Here's how the part is built. I have some questions about the finished solid (model axes, mm). A direction names the side the tool comes from. Give positions to 0.01 mm unless a question says otherwise; leave off trailing zeros. Loops run counter-clockwise (first coordinate to the right, second up) from the corner with the lowest first, then second, coordinate; pieces in that order, holes last. Notation, with made-up numbers: (2.25, 85) - (24.25, 85) arc R11 ccw to (24.25, 106) - close; hole circle Ø3 at (-39, -27.75). An arc over 180 degrees is marked (long way). Use a Markdown table: item, result.
from build123d import *

# Parameters (mm, degrees)
F0_W     = 10
F0_H     = 10.8
F1_DEPTH = 10
F2_R     = 4
F3_DEPTH = 30
F4_R     = 2
F5_DEPTH = 25


with BuildPart() as f1:
    # F0 (on Right) → F1 (new body)
    with BuildSketch(Plane.YZ):
        with Locations((16.265796, 5.4)):
            Rectangle(F0_W, F0_H)
    extrude(amount=F1_DEPTH)

    # F2 (on face) → F3 (join)
    with BuildSketch(Plane.YZ.offset(10)):
        with Locations((16.265796, 5.4)):
            Circle(F2_R)
    extrude(amount=F3_DEPTH)

    # F4 (on face) → F5 (cut)
    with BuildSketch(Plane.XZ.offset(-11.265796)):
        with Locations((5, 5.4)):
            Circle(F4_R)
    extrude(amount=-F5_DEPTH, mode=Mode.SUBTRACT)


solid = f1.part
(1) If I drill on line 1 (Z direction, x = 5, y = 18.5); line 2 (X direction, y = 14.75, z = 5.5); line 3 (Z direction, x = 16.5, y = 16.25), over which ranges is the centre line in solid material (lowest first)?
A:
| item | result |
|---|---|
| line 1 | 0 to 3.4, 7.4 to 10.8 |
| line 2 | 0 to 3, 7 to 40 |
| line 3 | 1.4 to 9.4 |
(2) We'd pull the mould along Z, two halves only. Please class faces 3 (the face through (2.7, 11.266, 5.3)), 4 (the face through (24.79, 20.08, 6.6)), 5 (the face through (3.526, 16.196, 6.752)): pulls with the +Z half, pulls with the -Z half, needs draft (parallel to the pull), parting line crosses it, or undercut.
A:
| item | result |
|---|---|
| face 3 | needs draft |
| face 4 | parting line crosses it |
| face 5 | undercut |
(3) Will these pins go through, and if not, where does the flat tip stop? pin 1 (6 mm diameter, centred on x = 33, y = 14.5, fed in from +Z); pin 2 (5 mm diameter, centred on x = 23, z = 2, fed in from -Y); pin 3 (3 mm diameter, centred on x = 24, y = 13, fed in from +Z).
A:
| item | result |
|---|---|
| pin 1 | z = 9.4 |
| pin 2 | y = 12.37 |
| pin 3 | z = 8.99 |
(4) Suppose I cut it at A-A on z = 5.4. Write out the boundary of the cut face in (x, y).
A:
| item | result |
|---|---|
| outline | (0, 11.27) - (3, 11.27) - (3, 21.27) - (0, 21.27) - close; (7, 11.27) - (10, 11.27) - (10, 12.27) - (40, 12.27) - (40, 20.27) - (10, 20.27) - (10, 21.27) - (7, 21.27) - close |
(5) Suppose I cut it at D-D on z = 9. Write out the boundary of the cut face in (x, y).
A:
| item | result |
|---|---|
| outline | (0, 11.27) - (10, 11.27) - (10, 14.52) - (40, 14.52) - (40, 18.01) - (10, 18.01) - (10, 21.27) - (0, 21.27) - close |
(6) On a 3-axis mill with a long thin cutter (end or side, diameter ignored), from which of +Z, -Z, +X, -X, +Y, -Y can I reach the whole of each face in a straight line? I mean faces 1 (the face through (0, 16, 5)), 2 (the face through (10, 13, 8)). Say none if no direction works.
A:
| item | result |
|---|---|
| face 1 | +Z, -Z, -X, +Y, -Y |
| face 2 | +X |
(7) Suppose I cut it at B-B on x = 5. Write out the boundary of the cut face in (y, z), plus the area to 3 significant figures.
A:
| item | result |
|---|---|
| outline | (11.27, 0) - (21.27, 0) - (21.27, 3.4) - (11.27, 3.4) - close; (11.27, 7.4) - (21.27, 7.4) - (21.27, 10.8) - (11.27, 10.8) - close |
| area | 68.0 mm2 |
(8) Suppose I cut it at C-C on y = 16.75. Write out the boundary of the cut face in (x, z).
A:
| item | result |
|---|---|
| outline | (0, 0) - (10, 0) - (10, 1.43) - (40, 1.43) - (40, 9.37) - (10, 9.37) - (10, 10.8) - (0, 10.8) - close; hole circle Ø4 at (5, 5.4) |
